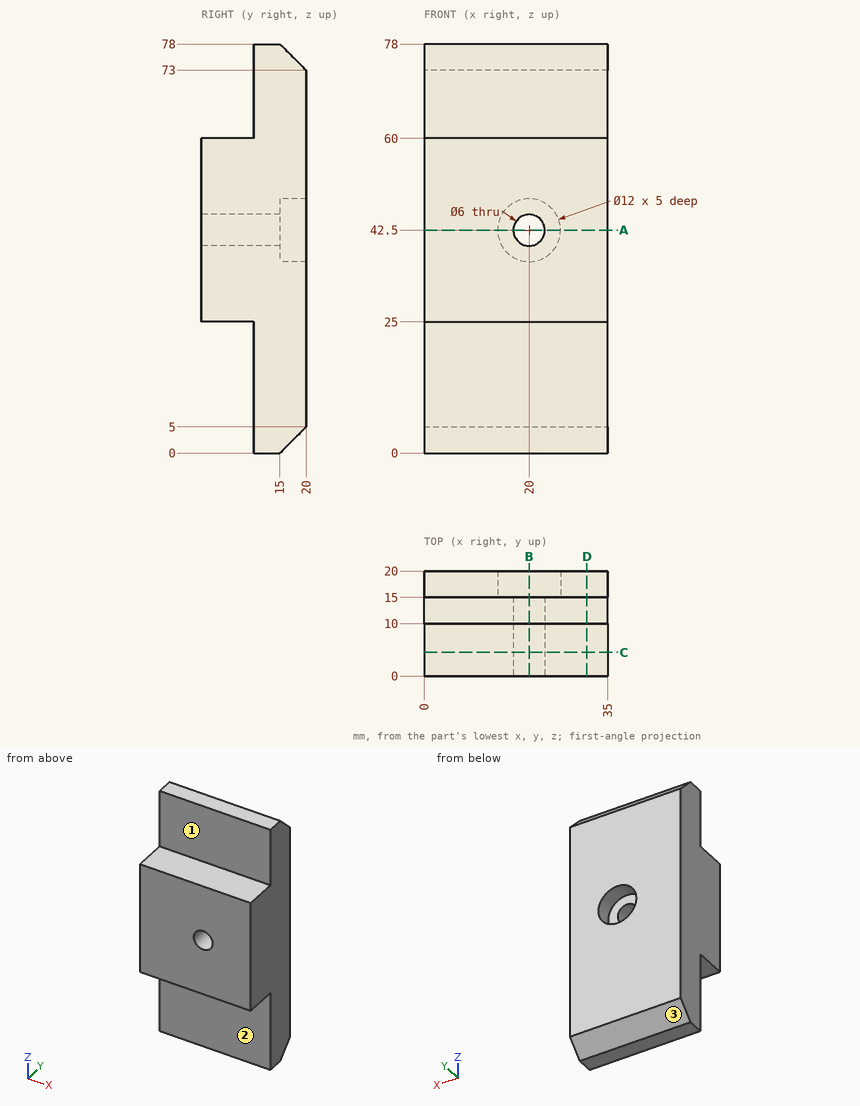
Verification items for this drawing (mm, ordinates from the low corner). A direction names the side the tool comes from. Round coordinates to 2 decimals unless told otherwise and drop trailing zeros. Write each loop counter-clockwise with the first axis right and the second up, starting at its lowest first coordinate (ties: lowest second). Pieces come first, ordered by that corner, then holes. Notation, with made-up numbers: (-2, 56.25) - (7, 56.25) arc R11 ccw to (7, 63.25) - close; hole circle Ø1 at (57.5, 1). An arc over 180 degrees is marked (long way). One line per item, written item: value.
1. Depth check by flat-ended pin: pin 1 Ø8 at (x, y) = (17.5, 4.5) entering from -Z; pin 2 Ø8 at (x, y) = (9, 3) entering from +Z; pin 3 Ø20 at (x, z) = (11.5, 10.5) entering from -Y. Enter the tip coordinate at first touch or a pass-through.
The answers:
pin 1: stops at z = 25
pin 2: stops at z = 60
pin 3: stops at y = 10
2. Cross-section at D-D on x = 31. Record the boundary of the cut face in (y, z).
The answers:
outline: (0, 25) - (10, 25) - (10, 0) - (15, 0) - (20, 5) - (20, 73) - (15, 78) - (10, 78) - (10, 60) - (0, 60) - close
3. Cross-section at B-B on x = 20. Record the boundary of the cut face in (y, z).
The answers:
outline: (0, 25) - (10, 25) - (10, 0) - (15, 0) - (20, 5) - (20, 36.5) - (15, 36.5) - (15, 39.5) - (0, 39.5) - close; (0, 45.5) - (15, 45.5) - (15, 48.5) - (20, 48.5) - (20, 73) - (15, 78) - (10, 78) - (10, 60) - (0, 60) - close
4. Set-up check for the marked faces 1, 2 and 3: record each of +Z, -Z, +X, -X, +Y, -Y from which the full face is reachable in a straight line by a thin tool's end or side.
The answers:
face 1: +Z, +X, -X, -Y
face 2: -Z, +X, -X, -Y
face 3: -Z, +X, -X, +Y
5. Cross-section at C-C on y = 4.5. Record the boundary of the cut face in (x, z), and give its area (3 significant figures).
The answers:
outline: (0, 25) - (35, 25) - (35, 60) - (0, 60) - close; hole circle Ø6 at (20, 42.5)
area: 1,200 mm^2
6. Scan lines: L1, parallel to X at y = 9.75, z = 42.5; L2, parallel to X at y = 18.5, z = 42.5; L3, parallel to Y at x = 20, z = 38. Record each from-to range of solid material in increasing order.
The answers:
L1: x = 0 to 17, 23 to 35
L2: x = 0 to 14, 26 to 35
L3: y = 0 to 15
7. Cross-section at A-A on z = 42.5. Record the boundary of the cut face in (x, y), and give its area (3 significant figures).
The answers:
outline: (0, 0) - (17, 0) - (17, 15) - (14, 15) - (14, 20) - (0, 20) - close; (23, 0) - (35, 0) - (35, 20) - (26, 20) - (26, 15) - (23, 15) - close
area: 550 mm^2
